```python
from build123d import *

# Parameters (mm, degrees)
F1_DEPTH   = 10.16
F2_SIZE2   = 8.89
F2_SIZE    = 6.35
F2_2_SIZE2 = 8.89
F2_2_SIZE  = 6.35
F2_3_SIZE2 = 8.89
F2_3_SIZE  = 6.35
F2_4_SIZE2 = 8.89
F2_4_SIZE  = 6.35


with BuildPart() as f1:
    # F0 (on Top) → F1 (new body)
    with BuildSketch(Plane.XY):
        with BuildLine():
            ThreePointArc((8.7829506919, -0.4383031513), (8.1984738627, -0.2271154175), (7.62, 0))
            ThreePointArc((7.62, 0), (7.3212709923, -2.1126739117), (6.4485062842, -4.0597003218))
            ThreePointArc((6.4485062842, -4.0597003218), (7.6729486494, -2.2858873029), (8.7829506919, -0.4383031513))
        make_face()
        with BuildLine():
            ThreePointArc((4.0597003218, 6.4485062842), (6.670806415, 3.6830343161), (7.62, 0))
            ThreePointArc((7.62, 0), (8.1984738627, -0.2271154175), (8.7829506919, -0.4383031513))
            ThreePointArc((8.7829506919, -0.4383031513), (11.6797251248, 6.4085522926), (13.0247462226, 13.7202996782))
            Line((13.0247462226, 13.7202996782), (1.3079377533, 20.32))
            ThreePointArc((1.3079377533, 20.32), (1.6208295824, 14.4951148577), (0.4383031513, 8.7829506919))
            ThreePointArc((0.4383031513, 8.7829506919), (2.2858873029, 7.6729486494), (4.0597003218, 6.4485062842))
        make_face()
        with BuildLine():
            ThreePointArc((0, 7.62), (2.1126739117, 7.3212709923), (4.0597003218, 6.4485062842))
            ThreePointArc((4.0597003218, 6.4485062842), (2.2858873029, 7.6729486494), (0.4383031513, 8.7829506919))
            ThreePointArc((0.4383031513, 8.7829506919), (0.2271154175, 8.1984738627), (0, 7.62))
        make_face()
        with BuildLine():
            ThreePointArc((8.7829506919, -0.4383031513), (7.6729486494, -2.2858873029), (6.4485062842, -4.0597003218))
            ThreePointArc((6.4485062842, -4.0597003218), (3.6830343161, -6.670806415), (0, -7.62))
            ThreePointArc((0, -7.62), (-0.2271154175, -8.1984738627), (-0.4383031513, -8.7829506919))
            ThreePointArc((-0.4383031513, -8.7829506919), (6.4085522926, -11.6797251248), (13.7202996782, -13.0247462226))
            Line((13.7202996782, -13.0247462226), (20.32, -1.3079377533))
            ThreePointArc((20.32, -1.3079377533), (14.4951148577, -1.6208295824), (8.7829506919, -0.4383031513))
        make_face()
        with BuildLine():
            ThreePointArc((-6.4485062842, 4.0597003218), (-3.6830343161, 6.670806415), (0, 7.62))
            ThreePointArc((0, 7.62), (0.2271154175, 8.1984738627), (0.4383031513, 8.7829506919))
            ThreePointArc((0.4383031513, 8.7829506919), (-6.4085522926, 11.6797251248), (-13.7202996782, 13.0247462226))
            Line((-13.7202996782, 13.0247462226), (-20.32, 1.3079377533))
            ThreePointArc((-20.32, 1.3079377533), (-14.4951148577, 1.6208295824), (-8.7829506919, 0.4383031513))
            ThreePointArc((-8.7829506919, 0.4383031513), (-7.6729486494, 2.2858873029), (-6.4485062842, 4.0597003218))
        make_face()
        with BuildLine():
            ThreePointArc((-0.4383031513, -8.7829506919), (-0.2271154175, -8.1984738627), (0, -7.62))
            ThreePointArc((0, -7.62), (-2.1126739117, -7.3212709923), (-4.0597003218, -6.4485062842))
            ThreePointArc((-4.0597003218, -6.4485062842), (-2.2858873029, -7.6729486494), (-0.4383031513, -8.7829506919))
        make_face()
        with BuildLine():
            ThreePointArc((-7.62, 0), (-7.3212709923, 2.1126739117), (-6.4485062842, 4.0597003218))
            ThreePointArc((-6.4485062842, 4.0597003218), (-7.6729486494, 2.2858873029), (-8.7829506919, 0.4383031513))
            ThreePointArc((-8.7829506919, 0.4383031513), (-8.1984738627, 0.2271154175), (-7.62, 0))
        make_face()
        with BuildLine():
            ThreePointArc((-0.4383031513, -8.7829506919), (-2.2858873029, -7.6729486494), (-4.0597003218, -6.4485062842))
            ThreePointArc((-4.0597003218, -6.4485062842), (-6.670806415, -3.6830343161), (-7.62, 0))
            ThreePointArc((-7.62, 0), (-8.1984738627, 0.2271154175), (-8.7829506919, 0.4383031513))
            ThreePointArc((-8.7829506919, 0.4383031513), (-11.6797251248, -6.4085522926), (-13.0247462226, -13.7202996782))
            Line((-13.0247462226, -13.7202996782), (-1.3079377533, -20.32))
            ThreePointArc((-1.3079377533, -20.32), (-1.6208295824, -14.4951148577), (-0.4383031513, -8.7829506919))
        make_face()
        with BuildLine():
            ThreePointArc((6.4485062842, -4.0597003218), (7.3212709923, -2.1126739117), (7.62, 0))
            ThreePointArc((7.62, 0), (6.670806415, 3.6830343161), (4.0597003218, 6.4485062842))
            ThreePointArc((4.0597003218, 6.4485062842), (2.1126739117, 7.3212709923), (0, 7.62))
            ThreePointArc((0, 7.62), (-3.6830343161, 6.670806415), (-6.4485062842, 4.0597003218))
            ThreePointArc((-6.4485062842, 4.0597003218), (-7.3212709923, 2.1126739117), (-7.62, 0))
            ThreePointArc((-7.62, 0), (-6.670806415, -3.6830343161), (-4.0597003218, -6.4485062842))
            ThreePointArc((-4.0597003218, -6.4485062842), (-2.1126739117, -7.3212709923), (0, -7.62))
            ThreePointArc((0, -7.62), (3.6830343161, -6.670806415), (6.4485062842, -4.0597003218))
        make_face()
    extrude(amount=F1_DEPTH)

    # F2
    f2_edges = [f1.edges().sort_by_distance(p)[0] for p in [
        (1.62083, 14.495115, 10.16),
    ]]
    f2_side = f1.faces().sort_by_distance((1.62083, 14.495115, 5.08))[0]
    chamfer(f2_edges, length=F2_SIZE, length2=F2_SIZE2, reference=f2_side)

    # F2#2
    f2_2_edges = [f1.edges().sort_by_distance(p)[0] for p in [
        (-14.495115, 1.62083, 10.16),
    ]]
    f2_2_side = f1.faces().sort_by_distance((-14.495115, 1.62083, 5.08))[0]
    chamfer(f2_2_edges, length=F2_2_SIZE, length2=F2_2_SIZE2, reference=f2_2_side)

    # F2#3
    f2_3_edges = [f1.edges().sort_by_distance(p)[0] for p in [
        (-1.62083, -14.495115, 10.16),
    ]]
    f2_3_side = f1.faces().sort_by_distance((-1.62083, -14.495115, 5.08))[0]
    chamfer(f2_3_edges, length=F2_3_SIZE, length2=F2_3_SIZE2, reference=f2_3_side)

    # F2#4
    f2_4_edges = [f1.edges().sort_by_distance(p)[0] for p in [
        (14.495115, -1.62083, 10.16),
    ]]
    f2_4_side = f1.faces().sort_by_distance((14.495115, -1.62083, 5.08))[0]
    chamfer(f2_4_edges, length=F2_4_SIZE, length2=F2_4_SIZE2, reference=f2_4_side)


solid = f1.part
```
Can you work these out from the model? Positions are in its coordinate system, mm. A direction names the side the tool comes from. Round coordinates to 2 decimals unless told otherwise and drop trailing zeros. Loops run counter-clockwise (first coordinate to the right, second up) from the corner with the lowest first, then second, coordinate; pieces in that order, holes last. Notation, with made-up numbers: M 9,82.5 L 30,82.5 A30 ccw 30,114.5 Z; hole C 37,-24 d3. An arc over 180 degrees is marked long. Write item = value, one per line. Start each with the question number.
(1) Suppose I cut it at B-B on z = 5.25. Write out the boundary of the cut face in (x, y), plus the area to 3 significant figures.
(2) I need wall thicknesses on line 1 along X through (y, z) = (9, 5.5); line 2 along Y through (x, z) = (10, 4.5); line 3 along Y through (x, z) = (-8.5, 7.25). Which ranges of each line are inside material? Lowest first, please.
(3) Which directions (+Z, -Z, +X, -X, +Y, -Y) give clear straight access to the entire face, cutting with the end or side of a thin tool? Please do faces 4 (the face through (0, 0, 10.16)), 5 (the face through (-11.25, 5.74, 7.03)), 6 (the face through (14.577, -1.627, 1.878)), 7 (the face through (11.014, 4.412, 6.138)), 8 (the face through (-11.014, -4.412, 6.138)).
(4) If we mould it in two halves opening along X, with no side actions, what happens to faces 1 (the face through (-4.412, 11.014, 6.138)), 2 (the face through (16.24, -8.55, 3.88)), 3 (the face through (-8.55, -16.24, 3.88))? For each: released by +X, released by -X, zero draft, split by the parting line, or undercut.
(5) Suppose I cut it at A-A on z = 1. Write out the boundary of the cut face in (x, y).
(6) I'm going to push flat-ended pins straight in: P1, Ø5, axis at y = -10.5, z = 6, coming from the +X side; P2, Ø1.5, axis at x = -11, z = 3, coming from the -Y side; P3, Ø4, axis at x = -14.5, y = -6, coming from the -Z side; P4, Ø3, axis at y = -6.5, z = 8.5, coming from the -X side. Where does each tip first touch, or does it pass through?
Answer block:
q1.outline = M -19.07,3.53 A24.71 cw -7.73,2.2 A34.12 ccw -13.02,-13.72 L -3.53,-19.07 A24.71 cw -2.2,-7.73 A34.12 ccw 13.72,-13.02 L 19.07,-3.53 A24.71 cw 7.73,-2.2 A34.12 ccw 13.02,13.72 L 3.53,19.07 A24.71 cw 2.2,7.73 A34.12 ccw -13.72,13.02 Z
q1.area = 666 mm²
q2.line_1 = -15.99 to 0.04, 2.99 to 12.35
q2.line_2 = -12.55 to -1.82, 1.96 to 15.42
q2.line_3 = -16.27 to 0.94, 5.4 to 12.23
q3.face_4 = +Z, +X, -X, +Y, -Y
q3.face_5 = +Z
q3.face_6 = +Z, -Z
q3.face_7 = +Z, +X
q3.face_8 = +Z, -X
q4.face_1 = undercut
q4.face_2 = released by +X
q4.face_3 = released by -X
q5.outline = M -20.32,1.31 A22.69 cw -8.78,0.44 A34.12 ccw -13.02,-13.72 L -1.31,-20.32 A22.69 cw -0.44,-8.78 A34.12 ccw 13.72,-13.02 L 20.32,-1.31 A22.69 cw 8.78,-0.44 A34.12 ccw 13.02,13.72 L 1.31,20.32 A22.69 cw 0.44,8.78 A34.12 ccw -13.72,13.02 Z
q6.P1 = 16.55
q6.P2 = -15.28
q6.P3 = through
q6.P4 = -12.11
